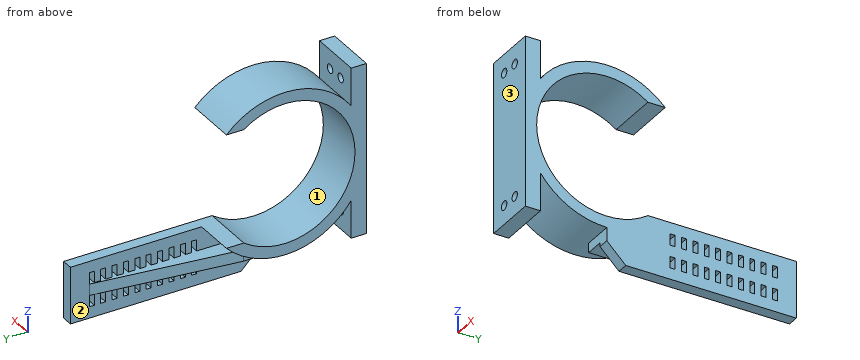
Autodesk Inventor part; units mm, degrees
ref_plane "YZ Plane" through (0, 0, 0) normal (1, 0, 0) x (0, 1, 0)
ref_plane "XZ Plane" through (0, 0, 0) normal (0, 1, 0) x (-1, 0, 0)
ref_plane "XY Plane" through (0, 0, 0) normal (0, 0, 1) x (1, 0, 0)
sketch "Sketch1" plane through (0, 0, 0) normal (1, 0, 0) x (0, 1, 0)
  circle A0 centre (0, 0) radius 23.495
  circle A1 centre (0, 0) radius 27.305
  line L0 (-27.305, 28.575) -> (-22.225, 28.575)
  line L1 (-22.225, 28.575) -> (-22.225, -28.575)
  line L2 (-22.225, -28.575) -> (-27.305, -28.575)
  line L3 (-27.305, -28.575) -> (-27.305, 28.575)
  line L4 (13.7518, 19.05) -> (13.7518, -19.05)
  line L5 (13.7518, 19.05) -> (19.5617, 19.05)
  line L6 (13.7518, -19.05) -> (19.5617, -19.05)
  point P0 (-22.225, 15.8623)
  point P1 (-22.225, -15.8623)
  dimension "d0" = 46.99
  dimension "d1" = 54.61
  dimension "d2" = 5.08
  dimension "d5" = 38.1
  dimension "d11" = 57.15
  dimension "d12" = 28.575
extrude "Extrusion1" add sketch "Sketch1" along normal blind 17.78 contours A0 L1 A1 L5 | L6 A1 L1 A0 | A0 L1 A1 | A1 L3 L0 L1 | L1 L2 L3 A1
sketch "Sketch2" plane through (17.78, 0, 0) normal (1, 0, 0) x (0, 0, -1)
  line L0 (19.05, 0) -> (38.1, 0)
  line L1 (38.1, 0) -> (38.1, 63.5)
  line L2 (38.1, 63.5) -> (19.05, 63.5)
  line L3 (19.05, 63.5) -> (19.05, 0)
  circle A0 centre (0, 0) radius 23.495
  circle A1 centre (0, 0) radius 27.305
  line L4 (19.05, 19.5617) -> (19.05, 13.7518)
  point P0 (19.05, 13.7518)
  point P1 (23.495, 0)
  dimension "d6" = 19.05
  dimension "d7" = 63.5
  dimension "d10" = 0
extrude "Extrusion2" add sketch "Sketch2" against normal blind 3.81 contours A0 L3 A1 L0 | A1 L3 L2 L1 L0 picked at (25.8542, 1.8052)
sketch "Sketch3" plane through (0, -27.305, -28.575) normal (0, -1, 0) x (1, 0, 0)
  circle A0 centre (11.8533, 50.8) radius 1.4986
  circle A1 centre (11.8533, 6.35) radius 1.4986
  line L0 (0, 57.15) -> (17.78, 57.15)
  line L1 (0, 0) -> (17.78, 0)
  line L2 (17.78, 57.15) -> (17.78, 0)
  circle A2 centre (5.9267, 6.35) radius 1.4986
  circle A3 centre (5.9267, 50.8) radius 1.4986
  line L3 (0, 57.15) -> (0, 0)
  point P0 (0, 28.575)
  dimension "d13" = 2.9972
  dimension "d14" = 2.9972
  dimension "d15" = 0
  dimension "d16" = 6.35
  dimension "d17" = 6.35
  dimension "d18" = 5.9267
  dimension "d32" = 2.9972
  dimension "d33" = 2.9972
  dimension "d34" = 5.9267
  dimension "d35" = 44.45
  dimension "d36" = 5.9267
extrude "Extrusion3" cut sketch "Sketch3" against normal blind 6.35 contours A0 | A1 | A2 | A3
sketch "Sketch4" plane through (13.97, 0, 0) normal (-1, 0, 0) x (0, 0, 1)
  line L0 (-30.48, 57.15) -> (-26.67, 57.15)
  line L1 (-26.67, 57.15) -> (-26.67, 0)
  line L2 (-26.67, 0) -> (-30.48, 0)
  line L3 (-30.48, 0) -> (-30.48, 57.15)
  line L4 (-38.1, 63.5) -> (-38.1, 0)
  line L5 (-19.05, 63.5) -> (-38.1, 63.5)
  line L6 (-38.1, 0) -> (-27.305, 0)
  point P0 (0, 0)
  dimension "d21" = 3.81
  dimension "d22" = 7.62
  dimension "d23" = 6.35
  dimension "d24" = 0
extrude "Extrusion4" add sketch "Sketch4" along normal blind 6.35
sketch "Sketch5" plane through (13.97, 0, -30.48) normal (0, 0, -1) x (-1, 0, 0)
  line L0 (0, 63.5) -> (0, 0)
  line L1 (0, 57.2597) -> (6.35, 9.3274)
  line L2 (6.35, 57.15) -> (6.35, 0)
  line L3 (-3.81, 0) -> (0, 0)
  line L4 (0, 0) -> (6.35, 0)
  line L5 (6.35, 0) -> (6.35, 57.15)
  line L6 (6.35, 57.15) -> (0, 57.15)
  line L7 (0, 57.15) -> (0, 0)
  point P0 (13.97, 0)
  point P1 (0.0145, 57.15)
extrude "Extrusion5" cut sketch "Sketch5" against normal blind 3.81 contours L6 L2 L1
chamfer "Chamfer1" distance 6.35 angle 45 1 edges at (15.875, 0, -38.1)
sketch "Sketch6" plane through (17.78, 0, 0) normal (1, 0, 0) x (0, 0, -1)
  line L0 (22.86, 57.15) -> (26.67, 57.15)
  line L1 (26.67, 57.15) -> (26.67, 55.499)
  line L2 (26.67, 55.499) -> (22.86, 55.499)
  line L3 (22.86, 55.499) -> (22.86, 57.15)
  line L4 (30.48, 57.15) -> (34.29, 57.15)
  line L5 (34.29, 57.15) -> (34.29, 55.499)
  line L6 (34.29, 55.499) -> (30.48, 55.499)
  line L7 (30.48, 55.499) -> (30.48, 57.15)
  line L8 (38.1, 63.5) -> (19.05, 63.5)
  line L9 (19.05, 63.5) -> (19.05, 13.7518)
  line L10 (38.1, 6.35) -> (38.1, 63.5)
  point P0 (0, 0)
  dimension "d37" = 1.651
  dimension "d38" = 6.35
  dimension "d39" = 3.81
  dimension "d40" = 3.81
  dimension "d41" = 3.81
  dimension "d42" = 3.81
  dimension "d43" = 3.81
extrude "Extrusion6" cut sketch "Sketch6" against normal blind 6.35
pattern_linear "Rectangular Pattern1" count 10 spacing 3.81 along (0, -1, 0) of "Extrusion6"
properties part number "LockMount"
The model under review builds one solid part; all positions refer to its coordinate system, in mm. Face numbers are marked on the shaded views. Give positions to 0.01 mm unless a question says otherwise; leave off trailing zeros. Loops run counter-clockwise (first coordinate to the right, second up) from the corner with the lowest first, then second, coordinate; pieces in that order, holes last. Notation, with made-up numbers: (-32, -15.5) - (21, -15.5) arc R32 cw to (21, 22.5) - close; hole circle Ø10 at (29, 65.5). An arc over 180 degrees is marked (long way). Answer as a JSON object with one key per item and string values.
Q1. To check wall thickness, follow line 1 along Z through (x, y) = (6.75, 0) (3 decimals); line 2 along X through (y, z) = (28.5, -21.5); line 3 along Z through (x, y) = (11.5, 0.5). State the ranges of each line that lie inside material, in increasing order.
Worked out:
{"line 1": "z = -27.305 to -23.495, 23.495 to 27.305", "line 2": "x = 13.97 to 17.78", "line 3": "z = -30.48 to -23.49, 23.49 to 27.3"}
Q2. Add section C-C on z = 0. State the section outline as (x, y) points (3 decimals), plus the area to 3 significant figures.
Worked out:
{"outline": "(0, -27.305) - (17.78, -27.305) - (17.78, -23.495) - (0, -23.495) - close", "area": "67.7 mm^2"}
Q3. Mouldability with a two-part tool opening along Y and no side actions: class the marked faces 1, 2 and 3 as +Y half, -Y half, draft (parallel to the pull), parting line (faces both ways), or undercut.
Worked out:
{"face 1": "undercut", "face 2": "draft", "face 3": "-Y half"}
Q4. Add section A-A on y = -13.5. State the section outline as (x, z) points.
Worked out:
{"outline": "(0, -23.73) - (17.78, -23.73) - (17.78, -19.23) - (0, -19.23) - close; (0, 19.23) - (17.78, 19.23) - (17.78, 23.73) - (0, 23.73) - close"}
Q5. Add section B-B on x = 6.25. State the section outline as (y, z) points (3 decimals), plus the area to 3 significant figures.
Worked out:
{"outline": "(-27.305, -28.575) - (-22.225, -28.575) - (-22.225, -23.688) - (-27.305, -23.688) - close; (-27.305, -20.762) - (-22.225, -20.762) - (-22.225, -15.862) arc R27.305 ccw to (19.562, -19.05) - (13.752, -19.05) arc R23.495 cw (long way) to (13.752, 19.05) - (19.562, 19.05) arc R27.305 ccw to (-22.225, 15.862) - (-22.225, 20.762) - (-27.305, 20.762) - close; (-27.305, 23.688) - (-22.225, 23.688) - (-22.225, 28.575) - (-27.305, 28.575) - close", "area": "595 mm^2"}
Q6. Insertion check: pin 1 (5.5 mm diameter, centred on y = 34, z = -30, fed in from -X); pin 2 (0.5 mm diameter, centred on x = 15.5, y = 33.5, fed in from +Z); pin 3 (1.5 mm diameter, centred on x = 6, z = 6.5, fed in from +Y). Each pin has a flat end and moves straight along its axis. Give the tip position at first contact, or say it passes through.
Worked out:
{"pin 1": "stops at x = 10.52", "pin 2": "stops at z = -19.05", "pin 3": "stops at y = -22.35"}
Q7. Add section D-D on y = 15. State the section outline as (x, z) points, plus the area to 3 significant figures.
Worked out:
{"outline": "(0, -22.82) - (13.97, -22.82) - (13.97, -26.67) - (8.37, -26.67) - (8.37, -30.48) - (13.97, -30.48) - (13.97, -38.1) - (17.78, -38.1) - (17.78, -19.05) - (0, -19.05) - close; (0, 19.05) - (17.78, 19.05) - (17.78, 22.82) - (0, 22.82) - close", "area": "213 mm^2"}
